Source: CAD feature listing. Evaluate the final solid. Frame: model axes, mm. A direction names the side the tool comes from. Coordinates: 2 decimals unless noted, no trailing zeros. Loops run counter-clockwise (first coordinate to the right, second up) from the corner with the lowest first, then second, coordinate; pieces in that order, holes last.
Item 1: Pin query (flat end, axial travel): pin 1 Ø7.5 at (x, z) = (-25.5, -2) entering from +Y; pin 2 Ø4.5 at (y, z) = (7, -2.5) entering from -X; pin 3 Ø2 at (y, z) = (6.5, 10.5) entering from -X. Return the tip coordinate at first contact, or that it passes through.
Item 2: Section query D-D, the plane z = 17.5. Return the cut outline in (x, y).
Item 3: Section query C-C, the plane x = 18. Return the cut outline in (y, z), then the cut area to 3 significant figures.
Item 4: Line query: probe 1 along X at (y, z) = (15, 1.5); probe 2 along X at (y, z) = (8, 16); probe 3 along Z at (x, y) = (-25.5, 15). Output: solid intervals per line, ascending.
Item 5: Section query B-B, the plane y = -6. Return the cut outline in (x, z), then the cut area to 3 significant figures.
Item 6: Pull-direction query (X, two-part tool) for faces 1 (the flat face through (30, 0, 0)), 2 (the flat face through (0, 12, 0)), 3 (the flat face through (0, 0, 20)), 4 (the flat face through (-20, 5, 10)); classes: +X half, -X half, draft (parallel to the pull), parting line (faces both ways), or undercut.
Item 7: Section query A-A, the plane z = -2. Return the cut outline in (x, y), then the cut area to 4 significant figures.
Item 8: Reachability of faces 5 (the flat face through (-15, 5, 0)), 6 (the flat face through (7, 5.5, 0)), 7 (the flat face through (25, 17.5, 0)) from +Z, -Z, +X, -X, +Y, -Y: full face, straight path, thin tool, end or side. Return the list, or none.
```python
from build123d import *

# Parameters (mm, degrees)
SKETCH_1_W          = 60
SKETCH_1_H          = 35
EXTRUDE_1_DEPTH     = 20
SKETCH_2_W          = 5
SKETCH_2_H          = 10
CUT_EXTRUDE_1_DEPTH = 25
SKETCH_3_W          = 5
SKETCH_3_H          = 8
CUT_EXTRUDE_2_DEPTH = 53.974050251


with BuildPart() as part:
    # Эскиз1 → Бобышка-Вытянуть1 (new, symmetric)
    with BuildSketch(Plane.XY):
        Rectangle(SKETCH_1_W, SKETCH_1_H)
    extrude(amount=EXTRUDE_1_DEPTH, both=True)

    # Эскиз2 → Вырез-Вытянуть1 (cut)
    with BuildSketch(Plane(origin=(0, 17.5, 0), x_dir=(1, 0, 0), z_dir=(0, 1, 0))):
        Polygon((-30, 15), (-30, -15), (-20, -15), (-20, -5), (-20, 5), (-20, 15), align=None)
        with Locations((-17.5, 0)):
            Rectangle(SKETCH_2_W, SKETCH_2_H)
    extrude(amount=-CUT_EXTRUDE_1_DEPTH, mode=Mode.SUBTRACT)

    # Эскиз3 → Вырез-Вытянуть2 (cut, through all)
    with BuildSketch(Plane.XY.offset(20)):
        Polygon((0, 17.5), (0, 5.5), (15, 5.5), (15, 9.5), (15, 17.5), align=None)
        with Locations((17.5, 13.5)):
            Rectangle(SKETCH_3_W, SKETCH_3_H)
    extrude(amount=-CUT_EXTRUDE_2_DEPTH, mode=Mode.SUBTRACT)


solid = part.part
```
Verdict:
1. pin 1: stops at y = -7.5
1. pin 2: stops at x = -15
1. pin 3: stops at x = -20
2. outline: (-30, -17.5) - (30, -17.5) - (30, 17.5) - (20, 17.5) - (20, 9.5) - (15, 9.5) - (15, 5.5) - (0, 5.5) - (0, 17.5) - (-30, 17.5) - close
3. outline: (-17.5, -20) - (9.5, -20) - (9.5, 20) - (-17.5, 20) - close
3. area: 1,080 mm2
4. probe 1: x = -15 to 0, 20 to 30
4. probe 2: x = -30 to 0, 15 to 30
4. probe 3: z = -20 to -15, 15 to 20
5. outline: (-30, -20) - (30, -20) - (30, 20) - (-30, 20) - (-30, 15) - (-20, 15) - (-20, 5) - (-15, 5) - (-15, -5) - (-20, -5) - (-20, -15) - (-30, -15) - close
5. area: 2,050 mm2
6. face 1: +X half
6. face 2: undercut
6. face 3: draft
6. face 4: -X half
7. outline: (-30, -17.5) - (30, -17.5) - (30, 17.5) - (20, 17.5) - (20, 9.5) - (15, 9.5) - (15, 5.5) - (0, 5.5) - (0, 17.5) - (-15, 17.5) - (-15, -7.5) - (-30, -7.5) - close
7. area: 1,505 mm2
8. face 5: -X, +Y
8. face 6: +Z, -Z, +Y
8. face 7: +Z, -Z, +X, -X, +Y
